Geometry check sheet. Reference: the model listing, model coordinates, mm. Face numbers are marked on the shaded views. Round coordinates to 2 decimals unless told otherwise and drop trailing zeros. Order: outer loops, then holes, each group sorted by start corner. A loop starts at its lowest first (then second) coordinate and runs counter-clockwise, first axis right, second up. Notation, with made-up numbers: (43, 79) - (65, 79) arc R11 cw to (65, 87) - close; hole circle Ø3 at (-2, -24.5). An arc over 180 degrees is marked (long way). One line per question, with ' | ' between items. Start each with the question number.
Q1. Mould release check, pull along Z, two halves, no side actions. Record for the marked faces 1, 2 and 3: +Z half, -Z half, draft (parallel to the pull), parting line (faces both ways), or undercut.
Q2. Sectioned sample at B-B, the plane y = 1.75. Enter the section's corners in (x, z).
Q3. Sectioned sample at C-C, the plane x = -59.5. Enter the section's corners in (y, z).
Q4. Sectioned sample at A-A, the plane y = 7.5. Enter the section's corners in (x, z).
Q5. Sectioned sample at D-D, the plane z = -27.5. Enter the section's corners in (x, y), then the cut area to 3 significant figures.
Q6. Material ranges on line 1 along Z through (x, y) = (1, -0.25); line 2 along X through (y, z) = (9.75, -43.5); line 3 along Z through (x, y) = (-5, 9.25), recorded low to high.
Q7. Gauge pin test, flat ends, axial feed: P1, Ø10, axis at y = -1, z = -12, coming from the -X side; P2, Ø5, axis at y = 0, z = -11.5, coming from the -X side; P3, Ø11.5, axis at x = -8.93, z = -35, coming from the -Y side. Record the tip position at first contact, or that the pin passes through.
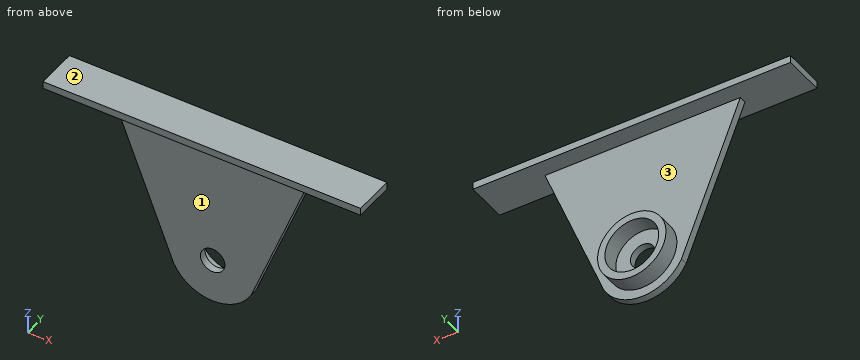
```python
from build123d import *

# Parameters (mm, degrees)
BOSS_EXTRUDE1_DEPTH = 3
SKETCH2_R           = 14
SKETCH2_R_2         = 11
BOSS_EXTRUDE2_DEPTH = 7
SKETCH3_W           = 130
SKETCH3_H           = 17
BOSS_EXTRUDE3_DEPTH = 3
SKETCH5_R           = 5
CUT_EXTRUDE1_DEPTH  = 10


with BuildPart() as part:
    # Sketch1 → Boss-Extrude1 (new body)
    with BuildSketch(Plane(origin=(0, 0, 0), x_dir=(1, 0, 0), z_dir=(0, 1, 0))):
        with BuildLine():
            Line((-48.929144451, -17.835062273), (31.070855549, -17.835062273))
            Line((31.070855549, -17.835062273), (6.985518971, 43.196988966))
            ThreePointArc((6.985518971, 43.196988966), (-8.929144451, 52.904273338), (-24.843807874, 43.196988966))
            Line((-24.843807874, 43.196988966), (-48.929144451, -17.835062273))
        make_face()
    extrude(amount=BOSS_EXTRUDE1_DEPTH)

    # Sketch2 → Boss-Extrude2 (add)
    with BuildSketch(Plane(origin=(0, 3, 0), x_dir=(1, 0, 0), z_dir=(0, 1, 0))):
        with Locations((-8.929144451, 35.004937727)):
            Circle(SKETCH2_R)
        with Locations((-8.929144451, 35.004937727)):
            Circle(SKETCH2_R_2, mode=Mode.SUBTRACT)
    extrude(amount=BOSS_EXTRUDE2_DEPTH)

    # Sketch3 → Boss-Extrude3 (add)
    with BuildSketch(Plane.XY.offset(17.835062273)):
        with Locations((-8.929144451, 1.5)):
            Rectangle(SKETCH3_W, SKETCH3_H)
    extrude(amount=BOSS_EXTRUDE3_DEPTH)

    # Sketch5 → Cut-Extrude1 (cut)
    with BuildSketch(Plane(origin=(0, 3, 0), x_dir=(1, 0, 0), z_dir=(0, 1, 0))):
        with Locations((-8.929144451, 35.004937727)):
            Circle(SKETCH5_R)
    extrude(amount=-CUT_EXTRUDE1_DEPTH, mode=Mode.SUBTRACT)


solid = part.part
```
Determined:
1) face 1: draft | face 2: +Z half | face 3: undercut
2) outline: (-73.93, 17.84) - (-48.93, 17.84) - (-24.84, -43.2) arc R17.9 ccw to (6.99, -43.2) - (31.07, 17.84) - (56.07, 17.84) - (56.07, 20.84) - (-73.93, 20.84) - close; hole circle Ø10 at (-8.93, -35)
3) outline: (-7, 17.84) - (10, 17.84) - (10, 20.84) - (-7, 20.84) - close
4) outline: (-73.93, 17.84) - (56.07, 17.84) - (56.07, 20.84) - (-73.93, 20.84) - close; circle Ø28 at (-8.93, -35); hole circle Ø22 at (-8.93, -35)
5) outline: (-31.04, 0) - (13.18, 0) - (13.18, 3) - (2.89, 3) - (2.89, 10) - (-0.89, 10) - (-0.89, 3) - (-16.97, 3) - (-16.97, 10) - (-20.75, 10) - (-20.75, 3) - (-31.04, 3) - close | area: 186 mm2
6) line 1: z = 17.84 to 20.84 | line 2: x = -20.06 to -15.92, -1.94 to 2.2 | line 3: z = -48.44 to -45.28, -24.73 to -21.57, 17.84 to 20.84
7) P1: stops at x = -39.09 | P2: stops at x = -38.34 | P3: stops at y = 0
